Autodesk Inventor part; units mm, degrees
ref_plane "YZ Plane" through (0, 0, 0) normal (1, 0, 0) x (0, 1, 0)
ref_plane "XZ Plane" through (0, 0, 0) normal (0, 1, 0) x (-1, 0, 0)
ref_plane "XY Plane" through (0, 0, 0) normal (0, 0, 1) x (1, 0, 0)
sketch "Sketch1" plane through (0, 0, 0) normal (0, 0, 1) x (1, 0, 0)
  line L0 (-290, -30) -> (290, -30)
  line L1 (290, -30) -> (290, 30)
  line L2 (290, 30) -> (-290, 30)
  line L3 (-290, 30) -> (-290, -30)
  line L4 (-290, -30) -> (290, 30) construction
  line L5 (290, -30) -> (-290, 30) construction
  line L6 (-100, 35) -> (100, 35)
  line L7 (100, 35) -> (100, 30)
  line L8 (100, 30) -> (-100, 30)
  line L9 (-100, 30) -> (-100, 35)
  line L10 (-100, 35) -> (100, 30) construction
  line L11 (100, 35) -> (-100, 30) construction
  line L12 (-290, 0) -> (290, 0)
  line L13 (-100, -35) -> (100, -35)
  line L14 (100, -35) -> (100, -30)
  line L15 (100, -30) -> (-100, -30)
  line L16 (-100, -30) -> (-100, -35)
  line L17 (-100, -35) -> (100, -30) construction
  line L18 (100, -35) -> (-100, -30) construction
  point P0 (0, 0)
  point P1 (0, 32.5)
  point P2 (0, 30)
  point P3 (0, -32.5)
  point P4 (0, -30)
  point P5 (-100, 30)
  point P6 (-100, -30)
  dimension "d0" = 580
  dimension "d1" = 60
  dimension "d2" = 5
  dimension "d3" = 200
extrude "Plate1" add sketch "Sketch1" along normal blind 5
equation "\"d4\" = Thickness"
equation "\"BendRadius\" = Thickness"
equation "\"BendReliefWidth\" = Thickness"
equation "\"BendReliefDepth\" = 0.5 * Thickness"
equation "\"TransitionRadius\" = BendRadius"
equation "\"JacobiRadiusSize\" = BendRadius"
equation "\"GapSize\" = Thickness"
properties part number "Table-Base Fixation"
For this review, take the finished solid that the model builds, in its own axes (mm). Coordinates: 2 decimals unless noted, no trailing zeros. Write each loop counter-clockwise with the first axis right and the second up, starting at its lowest first coordinate (ties: lowest second). Pieces come first, ordered by that corner, then holes. Notation, with made-up numbers: (37, 23) - (43, 23) arc R19 ccw to (43, 32) - close; hole circle Ø9 at (-11, 38). An arc over 180 degrees is marked (long way). Answer in a Markdown table with one row per item. Add a question column.
Q1. We need section A-A, the plane z = 1.75. State the section outline as (x, y) points.
Q2. For probe 1 along Y at (x, z) = (168, 1.1); probe 2 along X at (y, z) = (32, 1.85), list the stretches that pass through material, from the lowest coordinate up.
Q3. For P1, Ø1.5, axis at y = 32.5, z = 2.5, coming from the -X side; P2, Ø1.5, axis at x = -193, z = 3.5, coming from the +Y side; P3, Ø1.5, axis at x = -222, z = 2.5, coming from the -Y side, all flat-tipped, find the tip position at first contact; note any pin that passes through.
Q4. We need section B-B, the plane x = -252.5. State the section outline as (y, z) points.
Answer list:
| question | item | result |
|---|---|---|
| 1 | outline | (-290, -30) - (-100, -30) - (-100, -35) - (100, -35) - (100, -30) - (290, -30) - (290, 30) - (100, 30) - (100, 35) - (-100, 35) - (-100, 30) - (-290, 30) - close |
| 2 | probe 1 | y = -30 to 30 |
| 2 | probe 2 | x = -100 to 100 |
| 3 | P1 | stops at x = -100 |
| 3 | P2 | stops at y = 30 |
| 3 | P3 | stops at y = -30 |
| 4 | outline | (-30, 0) - (30, 0) - (30, 5) - (-30, 5) - close |
